from build123d import *

# Parameters (mm, degrees)
SKETCH1_W                                           = 134
SKETCH1_H                                           = 100
BOSS_EXTRUDE1_DEPTH                                 = 12
SKETCH2_R                                           = 41
CUT_EXTRUDE1_DEPTH                                  = 4
SKETCH3_R                                           = 15
CUT_EXTRUDE2_DEPTH                                  = 84.982140959
M4_CLEARANCE_HOLE1_D                                = 4.3
M4_CLEARANCE_HOLE1_DEPTH                            = 15
M4_CLEARANCE_HOLE1_TIP                              = 1.291850331
CBORE_FOR_M6_HEX_SOCKET_HEAD_CAP_SCREW1_D           = 6.6
CBORE_FOR_M6_HEX_SOCKET_HEAD_CAP_SCREW1_DEPTH       = 15
CBORE_FOR_M6_HEX_SOCKET_HEAD_CAP_SCREW1_CBORE_D     = 11
CBORE_FOR_M6_HEX_SOCKET_HEAD_CAP_SCREW1_CBORE_DEPTH = 6.4
CBORE_FOR_M6_HEX_SOCKET_HEAD_CAP_SCREW1_TIP         = 1.982840043


with BuildPart() as part:
    # Sketch1 → Boss-Extrude1 (new body)
    with BuildSketch(Plane(origin=(0, 0, 0), x_dir=(1, 0, 0), z_dir=(0, 1, 0))):
        Rectangle(SKETCH1_W, SKETCH1_H)
    extrude(amount=BOSS_EXTRUDE1_DEPTH)

    # Sketch2 → Cut-Extrude1 (cut)
    with BuildSketch(Plane(origin=(0, 12, 0), x_dir=(1, 0, 0), z_dir=(0, 1, 0))):
        with Locations(Location((0, 0, 0), (0, 0, 270))):
            Circle(SKETCH2_R)
    extrude(amount=-CUT_EXTRUDE1_DEPTH, mode=Mode.SUBTRACT)

    # Sketch3 → Cut-Extrude2 (cut, through all)
    with BuildSketch(Plane(origin=(0, 8, 0), x_dir=(1, 0, 0), z_dir=(0, 1, 0))):
        with Locations(Location((0, 0, 0), (0, 0, 270))):
            Circle(SKETCH3_R)
    extrude(amount=-CUT_EXTRUDE2_DEPTH, mode=Mode.SUBTRACT)

    # M4 Clearance Hole1
    with Locations(Plane(origin=(0, 0, 0), x_dir=(-1, 0, 0), z_dir=(0, -1, 0))):
        with Locations((-21.25, 0), (0, 21.25), (21.25, 0), (0, -21.25)):
            Hole(M4_CLEARANCE_HOLE1_D / 2, depth=M4_CLEARANCE_HOLE1_DEPTH)
            with Locations((0, 0, -(M4_CLEARANCE_HOLE1_DEPTH + M4_CLEARANCE_HOLE1_TIP / 2))):  # 118° drill point
                Cone(0, M4_CLEARANCE_HOLE1_D / 2, M4_CLEARANCE_HOLE1_TIP, mode=Mode.SUBTRACT)

    # CBORE for M6 Hex Socket Head Cap Screw1
    with Locations(Plane(origin=(0, 12, 0), x_dir=(1, 0, 0), z_dir=(0, 1, 0))):
        with Locations((59, 40), (-59, 40), (-59, 0), (-59, -40), (59, 0), (59, -40)):
            CounterBoreHole(CBORE_FOR_M6_HEX_SOCKET_HEAD_CAP_SCREW1_D / 2, CBORE_FOR_M6_HEX_SOCKET_HEAD_CAP_SCREW1_CBORE_D / 2, CBORE_FOR_M6_HEX_SOCKET_HEAD_CAP_SCREW1_CBORE_DEPTH, depth=CBORE_FOR_M6_HEX_SOCKET_HEAD_CAP_SCREW1_DEPTH)
            with Locations((0, 0, -(CBORE_FOR_M6_HEX_SOCKET_HEAD_CAP_SCREW1_DEPTH + CBORE_FOR_M6_HEX_SOCKET_HEAD_CAP_SCREW1_TIP / 2))):  # 118° drill point
                Cone(0, CBORE_FOR_M6_HEX_SOCKET_HEAD_CAP_SCREW1_D / 2, CBORE_FOR_M6_HEX_SOCKET_HEAD_CAP_SCREW1_TIP, mode=Mode.SUBTRACT)


solid = part.part
Here's how the part is built. I have some questions about the finished solid (model axes, mm). A direction names the side the tool comes from. Round coordinates to 2 decimals unless told otherwise and drop trailing zeros. Order: outer loops, then holes, each group sorted by start corner. A loop starts at its lowest first (then second) coordinate and runs counter-clockwise, first axis right, second up. Notation, with made-up numbers: (47.5, -23) -> (94.5, -23) arc R18 ccw to (94.5, 6) -> close; hole circle Ø8 at (-19, 81). An arc over 180 degrees is marked (long way). Return JSON: item names as keys, results as strings.
Q1. If we section it at A-A on y = 10.5: List the corners of the cut face in (x, z) for me.
Filled sheet:
{"outline": "(-67, -50) -> (67, -50) -> (67, 50) -> (-67, 50) -> close; hole circle Ø11 at (-59, -40); hole circle Ø11 at (-59, 0); hole circle Ø11 at (-59, 40); hole circle Ø82 at (0, 0); hole circle Ø11 at (59, -40); hole circle Ø11 at (59, 0); hole circle Ø11 at (59, 40)"}
Q2. For pin 1 Ø9 at (x, z) = (59, 0) entering from -Y; pin 2 Ø3.5 at (x, z) = (-58.5, 37.5) entering from +Y, each with a flat end and sliding along its axis, tell me the tip position at first contact or that it passes through.
Filled sheet:
{"pin 1": "stops at y = 0", "pin 2": "stops at y = 5.6"}
Q3. If we section it at B-B on x = 59: List the corners of the cut face in (y, z) for me, plus the area to 3 significant figures.
Filled sheet:
{"outline": "(0, -50) -> (12, -50) -> (12, -45.5) -> (5.6, -45.5) -> (5.6, -43.3) -> (0, -43.3) -> close; (0, -36.7) -> (5.6, -36.7) -> (5.6, -34.5) -> (12, -34.5) -> (12, -5.5) -> (5.6, -5.5) -> (5.6, -3.3) -> (0, -3.3) -> close; (0, 3.3) -> (5.6, 3.3) -> (5.6, 5.5) -> (12, 5.5) -> (12, 34.5) -> (5.6, 34.5) -> (5.6, 36.7) -> (0, 36.7) -> close; (0, 43.3) -> (5.6, 43.3) -> (5.6, 45.5) -> (12, 45.5) -> (12, 50) -> (0, 50) -> close", "area": "878 mm^2"}
Q4. If we mould it in two halves opening along Z, with no side actions, what happens to faces 3 (the flat face through (-1, 6, -50)), 4 (the flat face through (-16, 0, -1)), 5 (the cylindrical face through (53.505, 8.845, -40.242))? For each: released by +Z, released by -Z, zero draft, split by the parting line, or undercut.
Filled sheet:
{"face 3": "released by -Z", "face 4": "zero draft", "face 5": "undercut"}
Q5. If we section it at C-C on z = -21.25: List the corners of the cut face in (x, y) for me, plus the area to 3 significant figures.
Filled sheet:
{"outline": "(-67, 0) -> (-2.15, 0) -> (-2.15, 8) -> (-35.06, 8) -> (-35.06, 12) -> (-67, 12) -> close; (2.15, 0) -> (67, 0) -> (67, 12) -> (35.06, 12) -> (35.06, 8) -> (2.15, 8) -> close", "area": "1,290 mm^2"}
Q6. I need wall thicknesses on line 1 along Z through (x, y) = (-59, 7); line 2 along X through (y, z) = (7, 40); line 3 along X through (y, z) = (1.9, -40). Which ranges of each line are inside material? Lowest first, please. Write a range as from..to.
Filled sheet:
{"line 1": "z = -50..-45.5, -34.5..-5.5, 5.5..34.5, 45.5..50", "line 2": "x = -67..-64.5, -53.5..53.5, 64.5..67", "line 3": "x = -67..-62.3, -55.7..55.7, 62.3..67"}
Q7. Which directions (+Z, -Z, +X, -X, +Y, -Y) give clear straight access to the entire face, cutting with the end or side of a thin tool? Please do faces 1 (the flat face through (59, 5.6, -36)), 2 (the cylindrical face through (19.1, 4.06, -0.09)).
Filled sheet:
{"face 1": "+Y", "face 2": "+Y, -Y"}
Q8. If we section it at D-D on x = -21.25: List the corners of the cut face in (y, z) for me.
Filled sheet:
{"outline": "(0, -50) -> (12, -50) -> (12, -35.06) -> (8, -35.06) -> (8, -2.15) -> (0, -2.15) -> close; (0, 2.15) -> (8, 2.15) -> (8, 35.06) -> (12, 35.06) -> (12, 50) -> (0, 50) -> close"}
